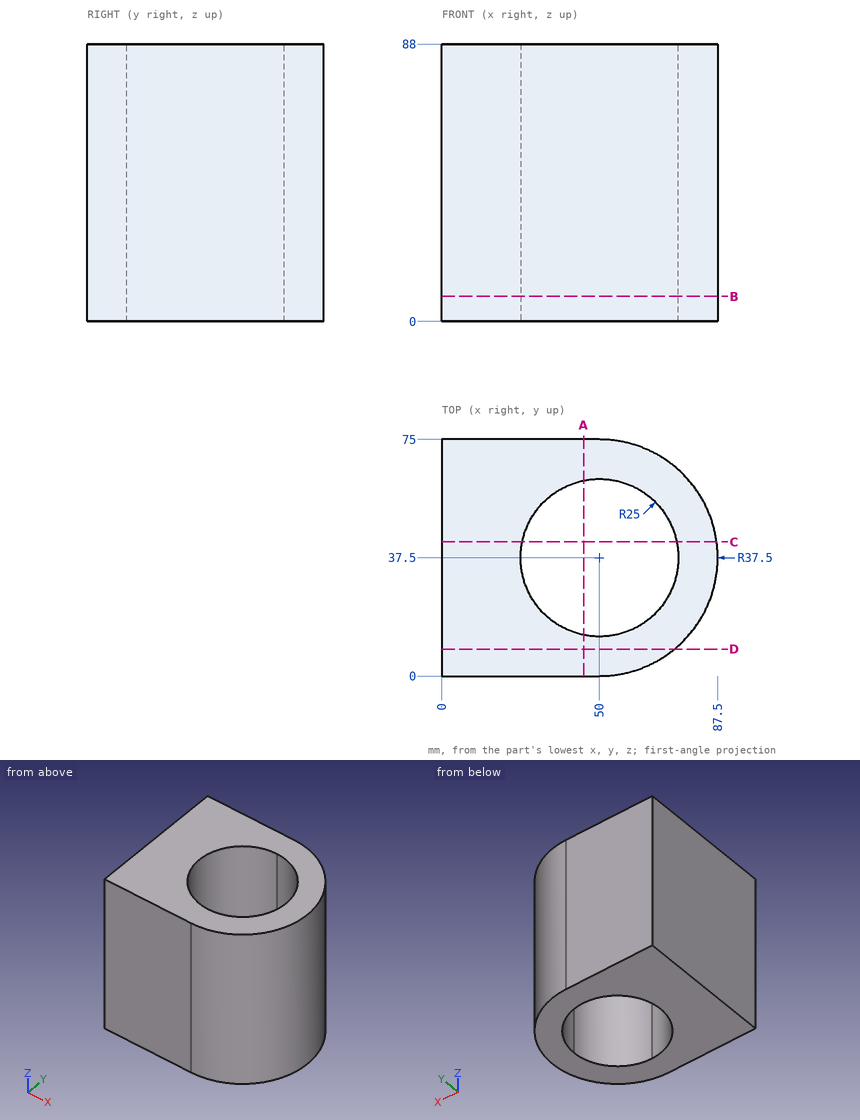
For this review, use the dimensioned drawing (mm, ordinates from the lowest corner) and the shaded views. Round coordinates to 2 decimals unless told otherwise and drop trailing zeros. Write each loop counter-clockwise with the first axis right and the second up, starting at its lowest first coordinate (ties: lowest second). Pieces come first, ordered by that corner, then holes. Notation, with made-up numbers: (27, 87) -> (42, 87) arc R6 cw to (42, 93) -> close; hole circle Ø5 at (-35, 56). An arc over 180 degrees is marked (long way). Use one line per item in the form item = value.
Q1. Consider section D-D (y = 8.5). State the section outline as (x, z) points (3 decimals), then the cut area to 3 significant figures.
Resolved:
outline = (0, 0) -> (73.775, 0) -> (73.775, 88) -> (0, 88) -> close
area = 6,490 mm²
Q2. Clearance check with flat-ended pins moving along their axes: pin 1 Ø1 at (y, z) = (22.5, 33) entering from +X; pin 2 Ø12 at (y, z) = (63, 37.5) entering from +X; pin 3 Ø12 at (y, z) = (59.5, 59.5) entering from +X. State where each tip first meets the part, or that it passes through.
Resolved:
pin_1 = 84.58
pin_2 = 82.03
pin_3 = 83.92
Q3. To check wall thickness, follow probe 1 along X at (y, z) = (37, 31.5) (3 decimals); probe 2 along Y at (x, z) = (50, 26.5); probe 3 along X at (y, z) = (54, 45). State the ranges of each line that lie inside material, in increasing order. Write a range as from..to.
Resolved:
probe_1 = 0..25.005, 74.995..87.497
probe_2 = 0..12.5, 62.5..75
probe_3 = 0..31.22, 68.78..83.67
Q4. Consider section B-B (z = 8). State the section outline as (x, y) points.
Resolved:
outline = (0, 0) -> (50, 0) arc R37.5 ccw to (50, 75) -> (0, 75) -> close; hole (50, 12.5) arc R25 ccw to (75, 37.5) arc R25 ccw to (50, 62.5) arc R25 ccw to start
Q5. Consider section C-C (y = 42.5). State the section outline as (x, z) points, then the cut area to 3 significant figures.
Resolved:
outline = (0, 0) -> (25.51, 0) -> (25.51, 88) -> (0, 88) -> close; (74.49, 0) -> (87.17, 0) -> (87.17, 88) -> (74.49, 88) -> close
area = 3,360 mm²
Q6. Consider section A-A (x = 45). State the section outline as (y, z) points, then the cut area to 3 significant figures.
Resolved:
outline = (0, 0) -> (13.01, 0) -> (13.01, 88) -> (0, 88) -> close; (61.99, 0) -> (75, 0) -> (75, 88) -> (61.99, 88) -> close
area = 2,290 mm²
